Autodesk Inventor part; units mm, degrees
ref_plane "EIS_XY" through (0, 0, 0) normal (0, 0, 1) x (1, 0, 0)
ref_plane "EIS_YZ" through (0, 0, 0) normal (1, 0, 0) x (0, 1, 0)
ref_plane "EIS_ZX" through (0, 0, 0) normal (0, 1, 0) x (0, 0, 1)
sketch "Sketch_1" plane through (0, 0, 0) normal (0, 0, 1) x (1, 0, 0)
  arc A0 (-11.2345, -6.1724) -> (-8.0966, -10) centre (-8.0966, -6.8) ccw
  line L0 (-8.0966, -10) -> (8.0966, -10)
  arc A1 (8.0966, -10) -> (11.2345, -6.1724) centre (8.0966, -6.8) ccw
  line L1 (11.2345, -6.1724) -> (8.8039, 5.9806)
  arc A2 (8.8039, 5.9806) -> (3.901, 10) centre (3.901, 5) ccw
  line L2 (3.901, 10) -> (-3.901, 10)
  arc A3 (-3.901, 10) -> (-8.8039, 5.9806) centre (-3.901, 5) ccw
  line L3 (-8.8039, 5.9806) -> (-11.2345, -6.1724)
extrude "Extrusion1" add sketch "Sketch_1" along normal blind 5
fillet "Fillet1" radius 3.2 8 edges at (-10.5713, -8.8288, 5) (0, -10, 5) (10.5713, -8.8288, 5) (10.0192, -0.0959, 5) (7.0709, 8.8667, 5) (0, 10, 5) (-7.0709, 8.8667, 5) (-10.0192, -0.0959, 5)
fillet "Fillet2" radius 0.5 8 edges at (-10.5713, -8.8288, 0) (-10.0192, -0.0959, 0) (-7.0709, 8.8667, 0) (0, 10, 0) (7.0709, 8.8667, 0) (10.0192, -0.0959, 0) (10.5713, -8.8288, 0) (0, -10, 0)
ref_plane "EIS_XY" through (0, 0, 0) normal (0, 0, 1) x (1, 0, 0)
ref_plane "EIS_YZ" through (0, 0, 0) normal (1, 0, 0) x (0, 1, 0)
ref_plane "EIS_ZX" through (0, 0, 0) normal (0, 1, 0) x (0, 0, 1)
properties part number "SCHUNK-1352153-Fingereinsatz Typ A Co-act EGP-C"
Work out the finished part from the listing and answer in its coordinate system (mm). Give positions to 0.01 mm unless a question says otherwise; leave off trailing zeros. Loops run counter-clockwise (first coordinate to the right, second up) from the corner with the lowest first, then second, coordinate; pieces in that order, holes last. Notation, with made-up numbers: (-21, 10) -> (-3, 10) arc R17 ccw to (-3, 25) -> close; hole circle Ø6 at (86.5, 29.5). An arc over 180 degrees is marked (long way). Write item = value, one per line. Start each with the question number.
(1) Find section B-B on z = 1.5. Give the vertices of the cut face in (x, y), and give its area (3 significant figures).
(2) Find section A-A on x = -1. Give the vertices of the cut face in (y, z).
(3) Find the intervals of material crossed by probe 1 along Y at (x, z) = (-4, 1.1); probe 2 along X at (y, z) = (-4.5, 3.9); probe 3 along Y at (x, z) = (8.5, 0.4), in increasing order. Write a range as from..to.
From the geometry:
q1.outline = (-11.23, -6.17) arc R3.2 ccw to (-8.1, -10) -> (8.1, -10) arc R3.2 ccw to (11.23, -6.17) -> (8.8, 5.98) arc R5 ccw to (3.9, 10) -> (-3.9, 10) arc R5 ccw to (-8.8, 5.98) -> close
q1.area = 386 mm^2
q2.outline = (-10, 0.5) arc R0.5 ccw to (-9.5, 0) -> (9.5, 0) arc R0.5 ccw to (10, 0.5) -> (10, 1.8) arc R3.2 ccw to (6.8, 5) -> (-6.8, 5) arc R3.2 ccw to (-10, 1.8) -> close
q3.probe_1 = -10..10
q3.probe_2 = -10.1..10.1
q3.probe_3 = -9.96..6.94
